Part model, mm, in its own coordinate system. Round coordinates to 2 decimals unless told otherwise and drop trailing zeros. Write each loop counter-clockwise with the first axis right and the second up, starting at its lowest first coordinate (ties: lowest second). Pieces come first, ordered by that corner, then holes. Notation, with made-up numbers: (40.25, 58.25) -> (96.25, 58.25) arc R15 ccw to (96.25, 85.25) -> close; hole circle Ø5 at (22, -0.75). An arc over 180 degrees is marked (long way). Return JSON: item names as keys, results as strings. Group by question number.
(1) Saw through at C-C (y = 10.75). List the corners of the cut face in (x, z), plus the area to 3 significant figures.
(2) Saw through at A-A (x = 0). List the corners of the cut face in (y, z), plus the area to 3 significant figures.
(3) Drill centre lines: L1, parallel to X at y = 8.4, z = 0; L2, parallel to Y at x = -5.5, z = -3; L3, parallel to Z at x = 1.5, y = 13. Where is each one in solid material? Low to high. Write a range as from..to.
(4) Saw through at B-B (z = 0). List the corners of the cut face in (x, y).
(5) Saw through at D-D (y = 5.75). List the corners of the cut face in (x, z), plus the area to 3 significant figures.
(6) Drop flat-ended pins along their axis: pin 1 Ø3 at (x, y) = (-9, 17.5) entering from -Z; pin 2 Ø4 at (y, z) = (5.5, 5) entering from -X; pin 3 Ø1.5 at (y, z) = (15.5, 10.5) entering from +X. Give the stop position or say it passes through.
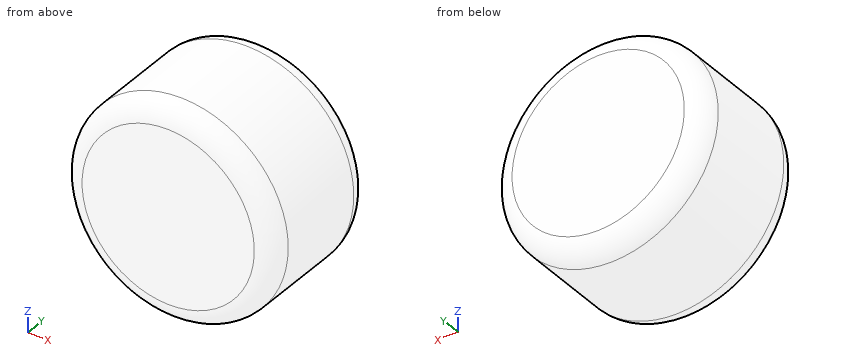
from build123d import *

# Parameters (mm, degrees)
SKETCH1_R           = 16
BOSS_EXTRUDE1_DEPTH = 20
SKETCH2_R           = 14.5
CUT_EXTRUDE1_DEPTH  = 18
BOSS_EXTRUDE2_START = -2
SKETCH3_R           = 16
BOSS_EXTRUDE2_DEPTH = 2
FILLET1_R           = 5
FILLET2_R           = 3


with BuildPart() as part:
    # Sketch1 → Boss-Extrude1 (new body)
    with BuildSketch(Plane(origin=(0, 0, 0), x_dir=(1, 0, 0), z_dir=(0, 1, 0))):
        with Locations(Location((0, 0, 0), (0, 0, 270))):
            Circle(SKETCH1_R)
    extrude(amount=BOSS_EXTRUDE1_DEPTH)

    # Sketch2 → Cut-Extrude1 (cut)
    with BuildSketch(Plane(origin=(0, 20, 0), x_dir=(1, 0, 0), z_dir=(0, 1, 0))):
        with Locations(Location((0, 0, 0), (0, 0, 270))):
            Circle(SKETCH2_R)
    extrude(amount=-CUT_EXTRUDE1_DEPTH, mode=Mode.SUBTRACT)

    # Sketch3 → Boss-Extrude2 (add)
    with BuildSketch(Plane(origin=(0, 20, 0), x_dir=(1, 0, 0), z_dir=(0, 1, 0)).offset(BOSS_EXTRUDE2_START)):
        with Locations(Location((0, 0, 0), (0, 0, 270))):
            Circle(SKETCH3_R)
    extrude(amount=BOSS_EXTRUDE2_DEPTH)

    # Fillet1
    fillet1_edges = [part.edges().sort_by_distance(p)[0] for p in [
        (0, 18, -14.5),
        (0, 2, -14.5),
    ]]
    fillet(fillet1_edges, radius=FILLET1_R)

    # Fillet2
    fillet2_edges = [part.edges().sort_by_distance(p)[0] for p in [
        (0, 0, -16),
        (0, 20, -16),
    ]]
    fillet(fillet2_edges, radius=FILLET2_R)


solid = part.part
Computed values:
{
 "1": {"outline": "circle Ø32 at (0, 0); hole circle Ø29 at (0, 0)", "area": "144 mm2"},
 "2": {"outline": "(0, -13) arc R3 ccw to (3, -16) -> (17, -16) arc R3 ccw to (20, -13) -> (20, 13) arc R3 ccw to (17, 16) -> (3, 16) arc R3 ccw to (0, 13) -> close; hole (2, -9.5) arc R5 ccw to (7, -14.5) -> (13, -14.5) arc R5 ccw to (18, -9.5) -> (18, 9.5) arc R5 ccw to (13, 14.5) -> (7, 14.5) arc R5 ccw to (2, 9.5) -> close", "area": "190 mm2"},
 "3": {"L1": "-16..-14.5, 14.5..16", "L2": "0..2, 18..20", "L3": "-15.93..-14.42, 14.42..15.93"},
 "4": {"outline": "(-16, 3) arc R3 ccw to (-13, 0) -> (13, 0) arc R3 ccw to (16, 3) -> (16, 17) arc R3 ccw to (13, 20) -> (-13, 20) arc R3 ccw to (-16, 17) -> close; hole (-14.5, 7) arc R5 ccw to (-9.5, 2) -> (9.5, 2) arc R5 ccw to (14.5, 7) -> (14.5, 13) arc R5 ccw to (9.5, 18) -> (-9.5, 18) arc R5 ccw to (-14.5, 13) -> close"},
 "5": {"outline": "circle Ø32 at (0, 0); hole circle Ø28.68 at (0, 0)", "area": "158 mm2"},
 "6": {"pin 1": "z = -14.11", "pin 2": "x = -15.72", "pin 3": "x = 12.69"}
}
